Build history of the part. All positions in model axes, mm. A direction names the side the tool comes from. Give positions to 0.01 mm unless a question says otherwise; leave off trailing zeros. Order: outer loops, then holes, each group sorted by start corner. A loop starts at its lowest first (then second) coordinate and runs counter-clockwise, first axis right, second up. Notation, with made-up numbers: M 32.5,3.5 L 47.5,3.5 A9 cw 47.5,11.5 Z; hole C 33,83 d4. An arc over 180 degrees is marked long. One line per item, written item: value. Start each with the question number.
from build123d import *

# Parameters (mm, degrees)
SKETCH1_W           = 25
SKETCH1_H           = 35
BOSS_EXTRUDE1_DEPTH = 8.2
SKETCH2_W           = 32
SKETCH2_H           = 6.7
CUT_EXTRUDE1_DEPTH  = 26
SKETCH3_W           = 30
SKETCH3_H           = 1.5
BOSS_EXTRUDE2_DEPTH = 5
SKETCH4_W           = 1.5
SKETCH4_H           = 30
BOSS_EXTRUDE3_DEPTH = 6.7
SKETCH5_W           = 30
SKETCH5_H           = 1.5
BOSS_EXTRUDE4_DEPTH = 5
SKETCH6_W           = 1.5
SKETCH6_H           = 30
BOSS_EXTRUDE5_DEPTH = 6.7
FILLET1_R           = 0.5
FILLET2_R           = 2


with BuildPart() as part:
    # Sketch1 → Boss-Extrude1 (new body)
    with BuildSketch(Plane(origin=(0, 6.7, 0), x_dir=(1, 0, 0), z_dir=(0, 1, 0))):
        Rectangle(SKETCH1_W, SKETCH1_H)
    extrude(amount=-BOSS_EXTRUDE1_DEPTH)

    # Sketch2 → Cut-Extrude1 (cut, through all)
    with BuildSketch(Plane(origin=(12.5, 0, 0), x_dir=(0, 0, -1), z_dir=(1, 0, 0))):
        with Locations((0, 3.35)):
            Rectangle(SKETCH2_W, SKETCH2_H)
    extrude(amount=-CUT_EXTRUDE1_DEPTH, mode=Mode.SUBTRACT)

    # Sketch3 → Boss-Extrude2 (add)
    with BuildSketch(Plane.ZY.offset(12.5)):
        with Locations((0, -0.75)):
            Rectangle(SKETCH3_W, SKETCH3_H)
    extrude(amount=BOSS_EXTRUDE2_DEPTH)

    # Sketch4 → Boss-Extrude3 (add)
    with BuildSketch(Plane.XZ.offset(1.5)):
        with Locations((-16.75, 0)):
            Rectangle(SKETCH4_W, SKETCH4_H)
    extrude(amount=BOSS_EXTRUDE3_DEPTH)

    # Sketch5 → Boss-Extrude4 (add)
    with BuildSketch(Plane(origin=(12.5, 0, 0), x_dir=(0, 0, -1), z_dir=(1, 0, 0))):
        with Locations((0, -0.75)):
            Rectangle(SKETCH5_W, SKETCH5_H)
    extrude(amount=BOSS_EXTRUDE4_DEPTH)

    # Sketch6 → Boss-Extrude5 (add)
    with BuildSketch(Plane.XZ.offset(1.5)):
        with Locations((16.75, 0)):
            Rectangle(SKETCH6_W, SKETCH6_H)
    extrude(amount=BOSS_EXTRUDE5_DEPTH)

    # Fillet1
    fillet1_edges = [part.edges().sort_by_distance(p)[0] for p in [
        (0, 0, -16),
        (0, 0, 16),
        (-16, -1.5, 0),
        (16, -1.5, 0),
    ]]
    fillet(fillet1_edges, radius=FILLET1_R)

    # Fillet2
    fillet2_edges = [part.edges().sort_by_distance(p)[0] for p in [
        (0, -1.5, -17.5),
        (-17.5, 0, 0),
        (0, -1.5, 17.5),
        (17.5, 0, 0),
    ]]
    fillet(fillet2_edges, radius=FILLET2_R)


solid = part.part
1) Slice it at B-B (z = 6). List the corners of the cut face in (x, y).
2) Drill centre lines: line 1 (X direction, y = -6.5, z = 4); line 2 (Y direction, x = 9, z = -14). Where is each one in solid material? Low to high.
3) Drop flat-ended pins along their axis: P1, Ø1, axis at x = 9, z = -9.5, coming from the -Y side; P2, Ø12, axis at x = -12, z = -3, coming from the +Y side; P3, Ø2.5, axis at x = 15, y = -2, coming from the -Z side; P4, Ø1.5, axis at x = -14.5, y = -4, coming from the +Z side. Give the stop position or say it passes through.
4) Pull direction Z, two halves, no side cores. Call faces 1 (the flat face through (-12.5, 3, 17)), 2 (the flat face through (0, 4, -17.5)), 3 (the flat face through (0, 4, -16)): pulls with the +Z half, pulls with the -Z half, needs draft (parallel to the pull), parting line crosses it, or undercut.
5) Slice it at A-A (y = -5). List the corners of the cut face in (x, z), plus the area to 3 significant figures.
6) Slice it at D-D (x = -10). List the corners of the cut face in (y, z).
7) Tool access for faces 4 (the flat face through (12.5, 3, -17)), 5 (the flat face through (-12.5, 3, -17)), 6 (the flat face through (16, -5, 0)), 7 (the flat face through (12.5, 3, 17)), 8 (the flat face through (0, 0, 0)): list every direction of +Z, -Z, +X, -X, +Y, -Y with a clear straight run to the whole face (end or side of a thin tool).
8) Slice it at C-C (y = 3.5). List the corners of the cut face in (x, z).
Results list:
1. outline: M -17.5,-8.2 L -16,-8.2 L -16,-2 A0.5 cw -15.5,-1.5 L 15.5,-1.5 A0.5 cw 16,-2 L 16,-8.2 L 17.5,-8.2 L 17.5,-2 A2 ccw 15.5,0 L -15.5,0 A2 ccw -17.5,-2 Z
2. line 1: x = -17.5 to -16, 16 to 17.5
2. line 2: y = -1.5 to 0
3. P1: stops at y = -1.5
3. P2: stops at y = 0
3. P3: stops at z = -15
3. P4: passes through
4. face 1: needs draft
4. face 2: pulls with the -Z half
4. face 3: undercut
5. outline: M -17.5,-15 L -16,-15 L -16,15 L -17.5,15 Z; M 16,-15 L 17.5,-15 L 17.5,15 L 16,15 Z
5. area: 90.0 mm²
6. outline: M -1.5,-15.5 A2 ccw 0.5,-17.5 L 6.7,-17.5 L 6.7,-16 L 0.5,-16 A0.5 cw 0,-15.5 L 0,15.5 A0.5 cw 0.5,16 L 6.7,16 L 6.7,17.5 L 0.5,17.5 A2 ccw -1.5,15.5 Z
7. face 4: -Z, +X, +Y, -Y
7. face 5: -Z, -X, +Y, -Y
7. face 6: +Z, -Z, -Y
7. face 7: +Z, +X, +Y, -Y
7. face 8: +X, -X, +Y
8. outline: M -12.5,-17.5 L 12.5,-17.5 L 12.5,-16 L -12.5,-16 Z; M -12.5,16 L 12.5,16 L 12.5,17.5 L -12.5,17.5 Z
